The figure shows three views and two pictorial views of one solid part (mm, origin at its lowest corner). Answer the questions. A direction names the side the tool comes from. Coordinates: 2 decimals unless noted, no trailing zeros. Loops run counter-clockwise (first coordinate to the right, second up) from the corner with the lowest first, then second, coordinate; pieces in that order, holes last. Notation, with made-up numbers: (10, 56.5) -> (24, 56.5) arc R16 ccw to (24, 66.5) -> close; hole circle Ø11 at (-2, -6.5). An arc over 180 degrees is marked (long way). Answer in a Markdown table with one row per item.
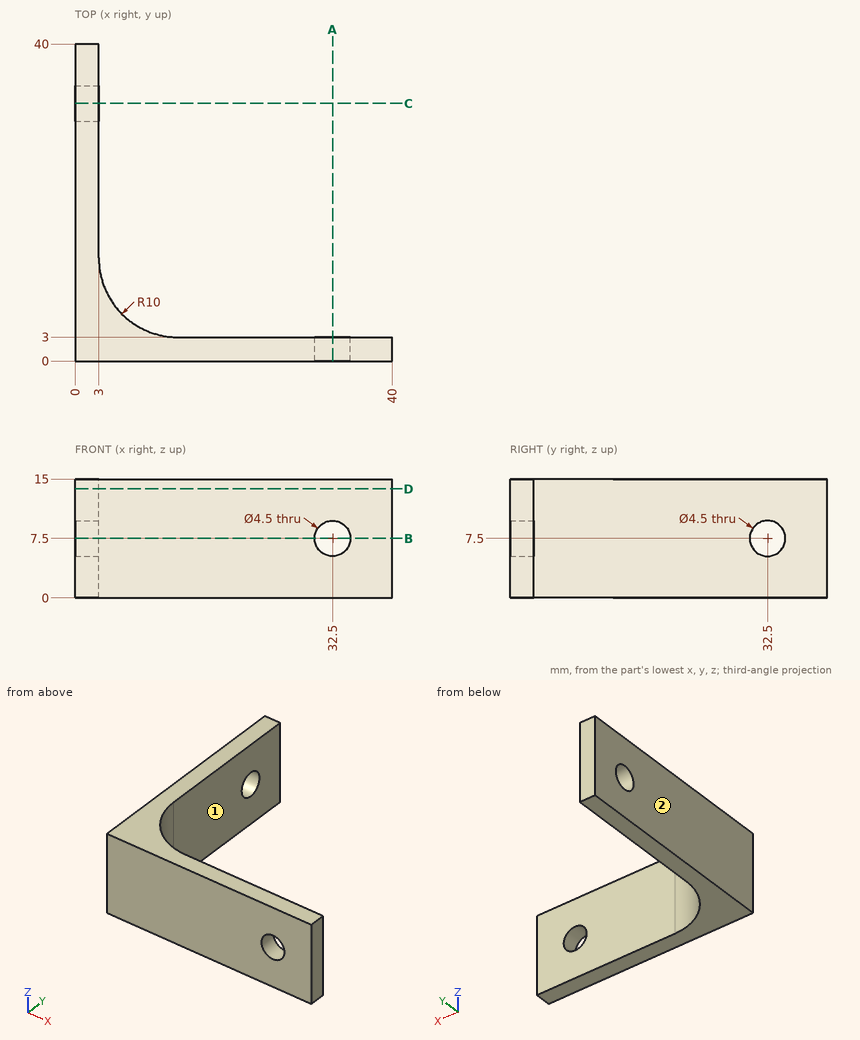
Item 1: A tool of negligible diameter and unlimited length cuts with its end or side. For the marked faces 1 and 2, from which of +Z, -Z, +X, -X, +Y, -Y can it reach the whole face along a straight path? Write none if from no direction.
Findings below:
| item | result |
|---|---|
| face 1 | +Z, -Z, +X, +Y |
| face 2 | +Z, -Z, -X, +Y, -Y |
Item 2: Find the intervals of material crossed by probe 1 along Z at (x, y) = (1.3, 32.5); probe 2 along X at (y, z) = (17, 6.5), in increasing order.
Findings below:
| item | result |
|---|---|
| probe 1 | z = 0 to 5.25, 9.75 to 15 |
| probe 2 | x = 0 to 3 |
Item 3: A cutting plane is placed at A-A, the plane x = 32.5. Determine the outline of the cut face in (y, z), plus the area to 3 significant figures.
Findings below:
| item | result |
|---|---|
| outline | (0, 0) -> (3, 0) -> (3, 5.25) -> (0, 5.25) -> close; (0, 9.75) -> (3, 9.75) -> (3, 15) -> (0, 15) -> close |
| area | 31.5 mm2 |
Item 4: A cutting plane is placed at B-B, the plane z = 7.5. Determine the outline of the cut face in (x, y), plus the area to 3 significant figures.
Findings below:
| item | result |
|---|---|
| outline | (0, 0) -> (30.25, 0) -> (30.25, 3) -> (13, 3) arc R10 cw to (3, 13) -> (3, 30.25) -> (0, 30.25) -> close; (0, 34.75) -> (3, 34.75) -> (3, 40) -> (0, 40) -> close; (34.75, 0) -> (40, 0) -> (40, 3) -> (34.75, 3) -> close |
| area | 225 mm2 |
Item 5: A cutting plane is placed at D-D, the plane z = 13.75. Determine the outline of the cut face in (x, y), plus the area to 3 significant figures.
Findings below:
| item | result |
|---|---|
| outline | (0, 0) -> (40, 0) -> (40, 3) -> (13, 3) arc R10 cw to (3, 13) -> (3, 40) -> (0, 40) -> close |
| area | 252 mm2 |
Item 6: Flat-ended cylindrical pins translate along their axes: pin 1 Ø7 at (y, z) = (32.5, 7.5) entering from +X; pin 2 Ø3.5 at (x, z) = (32.5, 7.5) entering from -Y; pin 3 Ø3 at (x, z) = (13.5, 1.5) entering from +Y. Find the tip coordinate at first contact, or state that the pin passes through.
Findings below:
| item | result |
|---|---|
| pin 1 | stops at x = 3 |
| pin 2 | passes through |
| pin 3 | stops at y = 3.05 |
